Input: part model. Units: mm. Frame: model coordinates. A direction names the side the tool comes from. Coordinates: 2 decimals unless noted, no trailing zeros. Order: outer loops, then holes, each group sorted by start corner. A loop starts at its lowest first (then second) coordinate and runs counter-clockwise, first axis right, second up. Notation, with made-up numbers: (-0.75, 26) -> (53.25, 26) arc R32 cw to (53.25, 53) -> close; hole circle Ø3 at (6, 18.5). An arc over 180 degrees is marked (long way). Answer as CSV lines item,"result".
from build123d import *

# Parameters (mm, degrees)
BOSS_EXTRU_1_DEPTH      = 45
ENL_V_MAT_EXTRU_1_DEPTH = 5
ESQUISSE4_W             = 37
ESQUISSE4_H             = 45
BOSS_EXTRU_2_DEPTH      = 5
ESQUISSE5_W             = 37
ESQUISSE5_H             = 10
BOSS_EXTRU_3_DEPTH      = 70
ESQUISSE6_R             = 1
ENL_V_MAT_EXTRU_2_DEPTH = 10
CHANFREIN2_SIZE         = 1
ESQUISSE7_W             = 12
ESQUISSE7_H             = 23
ENL_V_MAT_EXTRU_3_DEPTH = 10
ESQUISSE8_W             = 12
ESQUISSE8_H             = 5
ENL_V_MAT_EXTRU_4_DEPTH = 2.5
ESQUISSE10_R            = 1.5
ENL_V_MAT_EXTRU_5_DEPTH = 10


with BuildPart() as part:
    # Esquisse1 → Boss.-Extru.1 (new body)
    with BuildSketch(Plane.XY):
        Polygon((-40.10574777, 31.587127795), (-35.10574777, 31.587127795), (-35.10574777, -23.412872205), (-26.10574777, -23.412872205), (-26.10574777, -19.412872205), (-17.10574777, -19.412872205), (-17.10574777, -23.412872205), (-8.10574777, -23.412872205), (-8.10574777, 31.587127795), (-3.10574777, 31.587127795), (-3.10574777, -28.412872205), (-40.10574777, -28.412872205), align=None)
    extrude(amount=BOSS_EXTRU_1_DEPTH)

    # Esquisse2 → Enlèv. mat.-Extru.1 (cut)
    with BuildSketch(Plane(origin=(-3.10574777, 0, 0), x_dir=(0, 0, -1), z_dir=(1, 0, 0))):
        with BuildLine():
            Line((-12.5, 15.087127795), (-12.5, -9.912872205))
            ThreePointArc((-12.5, -9.912872205), (-22.5, -19.912872205), (-32.5, -9.912872205))
            Line((-32.5, -9.912872205), (-32.5, 15.087127795))
            ThreePointArc((-32.5, 15.087127795), (-22.5, 25.087127795), (-12.5, 15.087127795))
        make_face()
        with BuildLine():
            Line((-37.75, 9.877519714), (-37.75, -9.912872205))
            ThreePointArc((-37.75, -9.912872205), (-40, -12.162872205), (-42.25, -9.912872205))
            Line((-42.25, -9.912872205), (-42.25, 9.877519714))
            ThreePointArc((-42.25, 9.877519714), (-40, 12.127519714), (-37.75, 9.877519714))
        make_face()
        with BuildLine():
            Line((-2.75, 9.877519714), (-2.75, -10.122480286))
            ThreePointArc((-2.75, -10.122480286), (-5, -12.372480286), (-7.25, -10.122480286))
            Line((-7.25, -10.122480286), (-7.25, 9.877519714))
            ThreePointArc((-7.25, 9.877519714), (-5, 12.127519714), (-2.75, 9.877519714))
        make_face()
    extrude(amount=-ENL_V_MAT_EXTRU_1_DEPTH, mode=Mode.SUBTRACT)

    # Esquisse4 → Boss.-Extru.2 (add)
    with BuildSketch(Plane(origin=(0, 31.587127795, 0), x_dir=(1, 0, 0), z_dir=(0, 1, 0))):
        with Locations((-21.60574777, -22.5)):
            Rectangle(ESQUISSE4_W, ESQUISSE4_H)
    extrude(amount=BOSS_EXTRU_2_DEPTH)

    # Esquisse5 → Boss.-Extru.3 (add)
    with BuildSketch(Plane.XZ.offset(28.412872205)):
        with Locations((-21.60574777, 5)):
            Rectangle(ESQUISSE5_W, ESQUISSE5_H)
    extrude(amount=BOSS_EXTRU_3_DEPTH)

    # Esquisse6 → Enlèv. mat.-Extru.2 (cut)
    with BuildSketch(Plane.ZY.offset(40.10574777)):
        with Locations((15, -18.412872205)):
            Circle(ESQUISSE6_R)
        with Locations((15, -8.912872205)):
            Circle(ESQUISSE6_R)
    extrude(amount=-ENL_V_MAT_EXTRU_2_DEPTH, mode=Mode.SUBTRACT)

    # Chanfrein2
    chanfrein2_edges = [part.edges().sort_by_distance(p)[0] for p in [
        (-35.10574777, -18.412872205, 14),
        (-35.10574777, -8.912872205, 14),
    ]]
    chamfer(chanfrein2_edges, length=CHANFREIN2_SIZE)

    # Esquisse7 → Enlèv. mat.-Extru.3 (cut)
    with BuildSketch(Plane.XY.offset(10)):
        with Locations((-21.60574777, -72.912872205)):
            Rectangle(ESQUISSE7_W, ESQUISSE7_H)
    extrude(amount=-ENL_V_MAT_EXTRU_3_DEPTH, mode=Mode.SUBTRACT)

    # Esquisse8 → Enlèv. mat.-Extru.4 (cut)
    with BuildSketch(Plane.XY.offset(10)):
        with Locations((-21.60574777, -58.912872205)):
            Rectangle(ESQUISSE8_W, ESQUISSE8_H)
        with Locations((-21.60574777, -86.912872205)):
            Rectangle(ESQUISSE8_W, ESQUISSE8_H)
    extrude(amount=-ENL_V_MAT_EXTRU_4_DEPTH, mode=Mode.SUBTRACT)

    # Esquisse10 → Enlèv. mat.-Extru.5 (cut)
    with BuildSketch(Plane.XY.offset(10)):
        with Locations((-29.60574777, -35.912872205)):
            Circle(ESQUISSE10_R)
        with Locations((-29.60574777, -50.912872205)):
            Circle(ESQUISSE10_R)
        with Locations((-13.60574777, -50.912872205)):
            Circle(ESQUISSE10_R)
        with Locations((-13.60574777, -35.912872205)):
            Circle(ESQUISSE10_R)
    extrude(amount=-ENL_V_MAT_EXTRU_5_DEPTH, mode=Mode.SUBTRACT)


solid = part.part
1. Cut plane B-B (y = -80). Return the cut outline in (x, z), plus the area to 3 significant figures.
Findings:
outline,"(-40.11, 0) -> (-27.61, 0) -> (-27.61, 10) -> (-40.11, 10) -> close; (-15.61, 0) -> (-3.11, 0) -> (-3.11, 10) -> (-15.61, 10) -> close"
area,"250 mm2"
2. Ray query, line 1 along Y through (x, z) = (-26, 4.5); line 2 along Y through (x, z) = (-38.5, 15); line 3 along X through (y, z) = (-10.5, 33.5). Return the intervals inside material, ascending.
Findings:
line 1,"y = -98.41 to -84.41, -61.41 to -19.41, 31.59 to 36.59"
line 2,"y = -28.41 to -19.41, -17.41 to -9.91, -7.91 to 36.59"
line 3,"x = -40.11 to -35.11, -8.11 to -3.11"
3. Contact query for flat-ended pins moving along their axis: pin 1 (12 mm diameter, centred on x = -35.5, z = 28, fed in from -Y); pin 2 (5.5 mm diameter, centred on x = -23, y = -58, fed in from +Z); pin 3 (1 mm diameter, centred on y = -3.5, z = 27.5, fed in from +X). Output: stop coordinate, or through.
Findings:
pin 1,"stops at y = -28.41"
pin 2,"stops at z = 10"
pin 3,"stops at x = -35.11"
4. Mould query, pull axis Z, two halves, no side actions, for faces 1 (the face through (-31, -23.413, 22)), 2 (the face through (-6, 3, 12.5)), 3 (the face through (-6, 0, 42.25)), 4 (the face through (-22, -55, 10)). Classes: released by +Z, released by -Z, zero draft, split by the parting line, or undercut.
Findings:
face 1,"zero draft"
face 2,"undercut"
face 3,"undercut"
face 4,"released by +Z"
5. Cut plane C-C (z = 22.5). Return the cut outline in (x, y), plus the area to 3 significant figures.
Findings:
outline,"(-40.11, -28.41) -> (-3.11, -28.41) -> (-3.11, -19.91) -> (-8.11, -19.91) -> (-8.11, -23.41) -> (-17.11, -23.41) -> (-17.11, -19.41) -> (-26.11, -19.41) -> (-26.11, -23.41) -> (-35.11, -23.41) -> (-35.11, 31.59) -> (-8.11, 31.59) -> (-8.11, 25.09) -> (-3.11, 25.09) -> (-3.11, 36.59) -> (-40.11, 36.59) -> close"
area,"731 mm2"
6. Cut plane D-D (y = 22). Return the cut outline in (x, z), plus the area to 3 significant figures.
Findings:
outline,"(-40.11, 0) -> (-35.11, 0) -> (-35.11, 45) -> (-40.11, 45) -> close; (-8.11, 0) -> (-3.11, 0) -> (-3.11, 15.27) -> (-8.11, 15.27) -> close; (-8.11, 29.73) -> (-3.11, 29.73) -> (-3.11, 45) -> (-8.11, 45) -> close"
area,"378 mm2"
7. Reachability of faces 5 (the face through (-6, 2, 32.5)), 6 (the face through (-22, -59, 7.5)), 7 (the face through (-22, -84.413, 4)), 8 (the face through (-21, -28.413, 27)) from +Z, -Z, +X, -X, +Y, -Y: full face, straight path, thin tool, end or side. Return the list, or none.
Findings:
face 5,"+X"
face 6,"+Z"
face 7,"+Z, -Z"
face 8,"+Z, +X, -X, -Y"
8. Cut plane A-A (x = -9.5). Return the cut outline in (y, z), plus the area to 3 significant figures.
Findings:
outline,"(-98.41, 0) -> (-23.41, 0) -> (-23.41, 45) -> (-28.41, 45) -> (-28.41, 10) -> (-98.41, 10) -> close; (31.59, 0) -> (36.59, 0) -> (36.59, 45) -> (31.59, 45) -> close"
area,"1,150 mm2"
